The drawing under review shows one solid part. Ordinate dimensions are in mm from its lowest x, y, z. Give positions to 0.01 mm unless a question says otherwise; leave off trailing zeros. One line per item, written item: value. Start each with the question number.
1) Consider section A-A (z = 23.5). State how many separate pieces and enclosed holes the cut face has, plus the area to 3 significant figures.
2) Wall thickness on line 1 along Y through (x, z) = (41, 5.5) (1 decimal); line 2 along X through (y, z) = (83.5, 19) (1 decimal); line 3 along X through (y, z) = (28, 33) (1 decimal): over which ranges is each line inside the solid? List them lowest first. Write a range as from..to.
3) The part is to be moulded in two halves that separate along Y. For the marked faces 1, 2 and 3, say which applies: released by +Y, released by -Y, zero draft, split by the parting line, or undercut.
4) For pin 1 (5.5 mm diameter, centred on x = 73.28, y = 86.06, fed in from -Z); pin 2 (2 mm diameter, centred on y = 69, z = 18, fed in from -X) (1 decimal); pin 3 (2 mm diameter, centred on y = 21.5, z = 4.5, fed in from -X); pin 4 (4 mm diameter, centred on y = 52.5, z = 7, fed in from +X), all flat-tipped, find the tip position at first contact; note any pin that passes through.
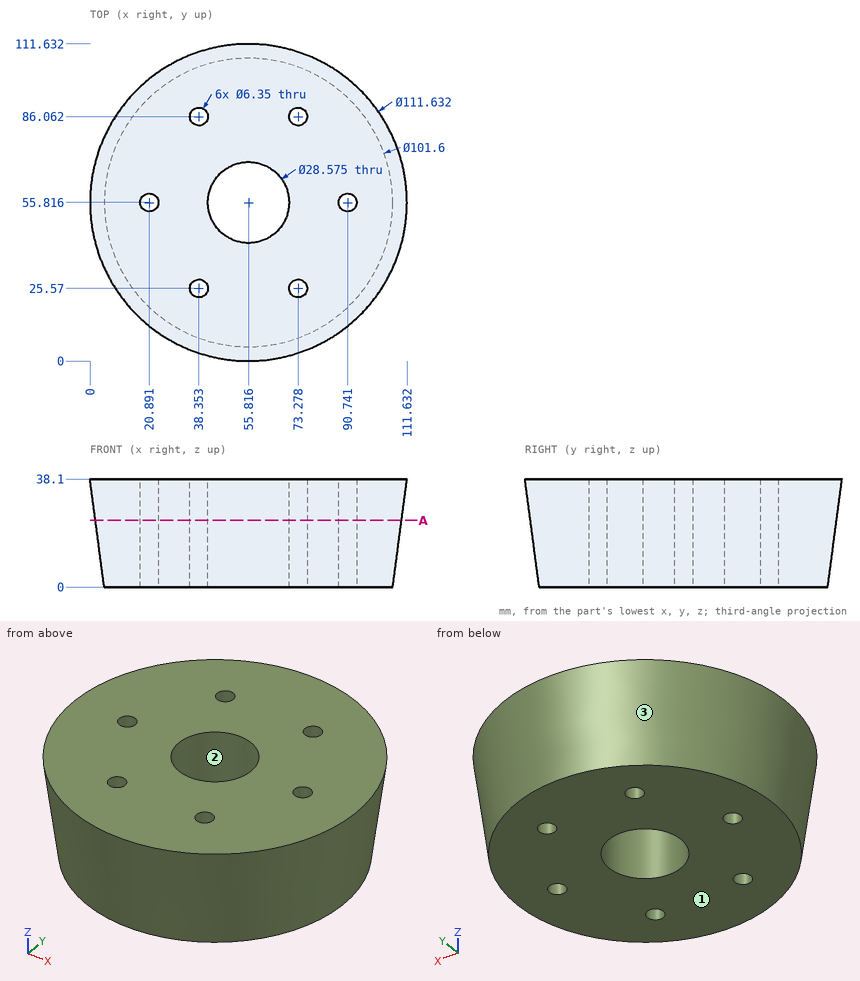
Checked values:
1. separate pieces: 1
1. enclosed holes: 7
1. area: 8,290 mm^2
2. line 1: y = 6.5..23.8, 27.3..84.3, 87.8..105.2
2. line 2: x = 10.3..36.5, 40.2..71.4, 75.2..101.4
2. line 3: x = 8.2..36.3, 40.4..71.2, 75.3..103.4
3. face 1: zero draft
3. face 2: undercut
3. face 3: split by the parting line
4. pin 1: passes through
4. pin 2: stops at x = 4
4. pin 3: stops at x = 16.67
4. pin 4: stops at x = 107.72
